Autodesk Inventor part; units mm, degrees
ref_plane "pad1_XY" through (-25.4, 0, 19.05) normal (1, 0, 0) x (0, 0, -1)
ref_plane "pad1_YZ" through (-25.4, 0, 19.05) normal (0, 0, -1) x (0, 1, 0)
ref_plane "pad1_ZX" through (-25.4, 0, 19.05) normal (0, 1, 0) x (1, 0, 0)
sketch "Sketch_1" plane through (0, 0, 0) normal (0, 0, 1) x (1, 0, 0)
  line L0 (-50.8, 30.988) -> (-50.8, 22.987)
  arc A0 (-50.8, 22.987) -> (-50.038, 22.225) centre (-50.038, 22.987) ccw
  line L1 (-50.038, 22.225) -> (-32.512, 22.225)
  arc A1 (-31.75, 21.463) -> (-32.512, 22.225) centre (-32.512, 21.463) ccw
  line L2 (-31.75, 21.463) -> (-31.75, -15.113)
  arc A2 (-31.75, -15.113) -> (-30.988, -15.875) centre (-30.988, -15.113) ccw
  line L3 (-30.988, -15.875) -> (-26.162, -15.875)
  arc A3 (-26.162, -15.875) -> (-25.4, -15.113) centre (-26.162, -15.113) ccw
  line L4 (-25.4, -15.113) -> (-25.4, 17.4498)
  line L5 (-25.4, 17.4498) -> (-17.4498, 25.4)
  line L6 (-17.4498, 25.4) -> (17.4498, 25.4)
  line L7 (17.4498, 25.4) -> (25.4, 17.4498)
  line L8 (25.4, 17.4498) -> (25.4, -15.113)
  arc A4 (25.4, -15.113) -> (26.162, -15.875) centre (26.162, -15.113) ccw
  line L9 (26.162, -15.875) -> (30.988, -15.875)
  arc A5 (30.988, -15.875) -> (31.75, -15.113) centre (30.988, -15.113) ccw
  line L10 (31.75, -15.113) -> (31.75, 21.463)
  arc A6 (32.512, 22.225) -> (31.75, 21.463) centre (32.512, 21.463) ccw
  line L11 (32.512, 22.225) -> (50.038, 22.225)
  arc A7 (50.038, 22.225) -> (50.8, 22.987) centre (50.038, 22.987) ccw
  line L12 (50.8, 22.987) -> (50.8, 30.988)
  arc A8 (50.8, 30.988) -> (50.038, 31.75) centre (50.038, 30.988) ccw
  line L13 (50.038, 31.75) -> (-50.038, 31.75)
  arc A9 (-50.038, 31.75) -> (-50.8, 30.988) centre (-50.038, 30.988) ccw
extrude "Extrusion1" add sketch "Sketch_1" along normal mid plane 71.4248
sketch "Sketch2" plane through (31.75, -15.113, 35.7124) normal (1, 0, 0) x (0, 0, -1)
  point P0 (16.6624, 15.113)
hole "Drilling 1" at (31.75, 0, 19.05) direction (-1, 0, 0) diameter 6.223 depth 63.5 countersink diameter 9.779 countersink angle 99.939
pattern_linear "Rectangular Pattern1" count 2 spacing 38.1 along (0, 0, -1) of "Drilling 1"
sketch "Sketch3" plane through (-50.038, 31.75, 35.7124) normal (0, 1, 0) x (1, 0, 0)
  point P0 (50.038, 16.6624)
hole "Drilling 2" at (0, 31.75, 19.05) direction (0, -1, 0) diameter 6.223 depth 6.35 countersink diameter 9.779 countersink angle 99.939
pattern_linear "Rectangular Pattern2" count 2 spacing 38.1 along (0, 0, -1) of "Drilling 2"
sketch "Sketch4" plane through (-50.038, 31.75, 35.7124) normal (0, 1, 0) x (1, 0, 0)
  point P0 (8.763, 16.6624)
hole "Drilling 3" at (-41.275, 31.75, 19.05) direction (0, -1, 0) diameter 8.3312 depth 9.525
pattern_linear "Rectangular Pattern3" count 2 spacing 82.55 along (1, 0, 0) count 2 spacing 38.1 along (0, 0, -1) of "Drilling 3"
ref_plane "pad1_XY" through (-25.4, 0, 19.05) normal (1, 0, 0) x (0, 0, -1)
ref_plane "pad1_YZ" through (-25.4, 0, 19.05) normal (0, 0, -1) x (0, 1, 0)
ref_plane "pad1_ZX" through (-25.4, 0, 19.05) normal (0, 1, 0) x (1, 0, 0)
ref_plane "pad2_XY" through (25.4, 0, 19.05) normal (1, 0, 0) x (0, 0, -1)
ref_plane "pad2_YZ" through (25.4, 0, 19.05) normal (0, 0, -1) x (0, 1, 0)
ref_plane "pad2_ZX" through (25.4, 0, 19.05) normal (0, 1, 0) x (1, 0, 0)
ref_plane "pad3_XY" through (0, 25.4, 19.05) normal (0, 1, 0) x (1, 0, 0)
ref_plane "pad3_YZ" through (0, 25.4, 19.05) normal (1, 0, 0) x (0, 0, -1)
ref_plane "pad3_ZX" through (0, 25.4, 19.05) normal (0, 0, -1) x (0, 1, 0)
ref_plane "s1_1_XY" through (-30.2565, 0, 19.05) normal (1, 0, 0) x (0, 0, -1)
ref_plane "s1_1_YZ" through (-30.2565, 0, 19.05) normal (0, 0, -1) x (0, 1, 0)
ref_plane "s1_1_ZX" through (-30.2565, 0, 19.05) normal (0, 1, 0) x (1, 0, 0)
ref_plane "s1_2_XY" through (-30.2565, 0, -19.05) normal (1, 0, 0) x (0, 0, -1)
ref_plane "s1_2_YZ" through (-30.2565, 0, -19.05) normal (0, 0, -1) x (0, 1, 0)
ref_plane "s1_2_ZX" through (-30.2565, 0, -19.05) normal (0, 1, 0) x (1, 0, 0)
ref_plane "s2_1_XY" through (30.2565, 0, 19.05) normal (1, 0, 0) x (0, 0, -1)
ref_plane "s2_1_YZ" through (30.2565, 0, 19.05) normal (0, 0, -1) x (0, 1, 0)
ref_plane "s2_1_ZX" through (30.2565, 0, 19.05) normal (0, 1, 0) x (1, 0, 0)
ref_plane "s2_2_XY" through (30.2565, 0, -19.05) normal (1, 0, 0) x (0, 0, -1)
ref_plane "s2_2_YZ" through (30.2565, 0, -19.05) normal (0, 0, -1) x (0, 1, 0)
ref_plane "s2_2_ZX" through (30.2565, 0, -19.05) normal (0, 1, 0) x (1, 0, 0)
ref_plane "s3_1_XY" through (0, 30.2565, 19.05) normal (0, 1, 0) x (1, 0, 0)
ref_plane "s3_1_YZ" through (0, 30.2565, 19.05) normal (1, 0, 0) x (0, 0, -1)
ref_plane "s3_1_ZX" through (0, 30.2565, 19.05) normal (0, 0, -1) x (0, 1, 0)
ref_plane "s3_2_XY" through (0, 30.2565, -19.05) normal (0, 1, 0) x (1, 0, 0)
ref_plane "s3_2_YZ" through (0, 30.2565, -19.05) normal (1, 0, 0) x (0, 0, -1)
ref_plane "s3_2_ZX" through (0, 30.2565, -19.05) normal (0, 0, -1) x (0, 1, 0)
properties part number "6835_p" material "Aluminum 6061"
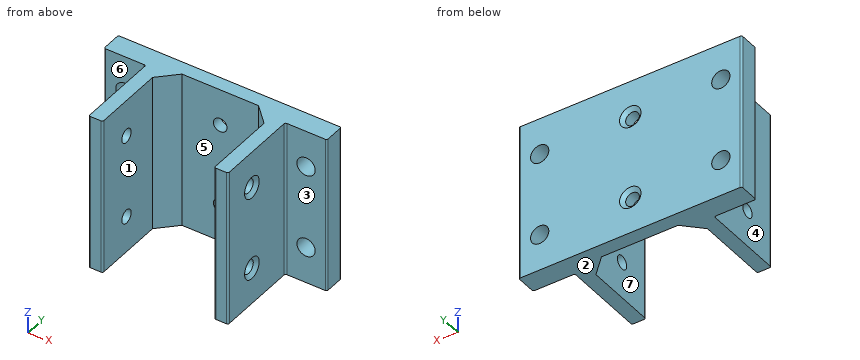
Read the model definition and answer for the solid it produces. Units are mm, in the model's axes. Face numbers are marked on the shaded views. A direction names the side the tool comes from. Coordinates: 2 decimals unless noted, no trailing zeros. Loops run counter-clockwise (first coordinate to the right, second up) from the corner with the lowest first, then second, coordinate; pieces in that order, holes last. Notation, with made-up numbers: (45, -18.5) -> (59, -18.5) arc R16 cw to (59, -13.5) -> close; hole circle Ø9 at (-40, 5). An arc over 180 degrees is marked (long way). Return JSON: item names as keys, results as strings.
Item 1: Find the intervals of material crossed by probe 1 along X at (y, z) = (27, -19); probe 2 along Z at (x, y) = (28, 0); probe 3 along X at (y, z) = (13, -31), in increasing order.
Answers:
{"probe 1": "x = -50.8 to -45.44, -37.11 to -3.11, 3.11 to 37.11, 45.44 to 50.8", "probe 2": "z = -35.71 to -22.16, -15.94 to 15.94, 22.16 to 35.71", "probe 3": "x = -31.75 to -25.4, 25.4 to 31.75"}
Item 2: For the marked faces 1, 2 and 3, determine the directions among +Z, -Z, +X, -X, +Y, -Y from which every point of the face is accessible in a straight line to the end or side of a thin tool.
Answers:
{"face 1": "+Z, -Z, -Y", "face 2": "-Z, +X, -X, +Y, -Y", "face 3": "+Z, -Z, +X, -Y"}
Item 3: Find section A-A (y = 0). Determine the outline of the cut face in (x, z), plus the area to 3 significant figures.
Answers:
{"outline": "(-31.75, -35.71) -> (-25.4, -35.71) -> (-25.4, -22.16) -> (-31.75, -22.16) -> close; (-31.75, -15.94) -> (-25.4, -15.94) -> (-25.4, 15.94) -> (-31.75, 15.94) -> close; (-31.75, 22.16) -> (-25.4, 22.16) -> (-25.4, 35.71) -> (-31.75, 35.71) -> close; (25.4, -35.71) -> (31.75, -35.71) -> (31.75, -23.94) -> (30.26, -22.16) -> (25.4, -22.16) -> close; (25.4, -15.94) -> (30.26, -15.94) -> (31.75, -14.16) -> (31.75, 14.16) -> (30.26, 15.94) -> (25.4, 15.94) -> close; (25.4, 22.16) -> (30.26, 22.16) -> (31.75, 23.94) -> (31.75, 35.71) -> (25.4, 35.71) -> close", "area": "744 mm2"}
Item 4: For a pull along X with two mould halves and no side action, classify the marked faces 4, 5, 6 and 7 as +X half, -X half, draft (parallel to the pull), parting line (faces both ways), or undercut.
Answers:
{"face 4": "-X half", "face 5": "undercut", "face 6": "draft", "face 7": "undercut"}
Item 5: Find section C-C (z = 27). Determine the outline of the cut face in (x, y) (3 decimals).
Answers:
{"outline": "(-50.8, 22.987) arc R0.762 ccw to (-50.038, 22.225) -> (-32.512, 22.225) arc R0.762 cw to (-31.75, 21.463) -> (-31.75, -15.113) arc R0.762 ccw to (-30.988, -15.875) -> (-26.162, -15.875) arc R0.762 ccw to (-25.4, -15.113) -> (-25.4, 17.45) -> (-17.45, 25.4) -> (17.45, 25.4) -> (25.4, 17.45) -> (25.4, -15.113) arc R0.762 ccw to (26.162, -15.875) -> (30.988, -15.875) arc R0.762 ccw to (31.75, -15.113) -> (31.75, 21.463) arc R0.762 cw to (32.512, 22.225) -> (50.038, 22.225) arc R0.762 ccw to (50.8, 22.987) -> (50.8, 30.988) arc R0.762 ccw to (50.038, 31.75) -> (-50.038, 31.75) arc R0.762 ccw to (-50.8, 30.988) -> close"}
Item 6: Flat-ended cylindrical pins translate along their axes: P1, Ø10, axis at y = 0, z = 19.05, coming from the +X side; P2, Ø8, axis at y = 0, z = -19.05, coming from the +X side; P3, Ø10, axis at y = -5, z = 12.5, coming from the -X side. Find the tip coordinate at first contact, or state that the pin passes through.
Answers:
{"P1": "stops at x = 31.75", "P2": "stops at x = 31", "P3": "stops at x = -31.75"}
Item 7: Find section B-B (x = 0). Determine the outline of the cut face in (y, z).
Answers:
{"outline": "(25.4, -35.71) -> (31.75, -35.71) -> (31.75, -23.94) -> (30.26, -22.16) -> (25.4, -22.16) -> close; (25.4, -15.94) -> (30.26, -15.94) -> (31.75, -14.16) -> (31.75, 14.16) -> (30.26, 15.94) -> (25.4, 15.94) -> close; (25.4, 22.16) -> (30.26, 22.16) -> (31.75, 23.94) -> (31.75, 35.71) -> (25.4, 35.71) -> close"}
Item 8: Find section D-D (x = -27.5). Count the separate pieces of the cut face and the enclosed holes in it, plus the area to 3 significant figures.
Answers:
{"separate pieces": "1", "enclosed holes": "2", "area": "3,340 mm2"}
